```python
from build123d import *

# Parameters (mm, degrees)
F1_DEPTH       = 6.35
F2_R           = 3.81
F3_DEPTH       = 6.35
F5_D           = 1.9304
F5_CSINK_D     = 4.2672
F5_CSINK_ANGLE = 82
F7_D           = 2.032


with BuildPart() as f1:
    # F0 (on Front) → F1 (new body)
    with BuildSketch(Plane.XZ):
        with BuildLine():
            ThreePointArc((-5.08, 12.7), (-3.5921024484, 9.1078975516), (0, 7.62))
            Line((0, 7.62), (0, 12.7))
            Line((0, 12.7), (0, 17.78))
            ThreePointArc((0, 17.78), (-3.5921024484, 16.2921024484), (-5.08, 12.7))
        make_face()
        with BuildLine():
            Line((0, 12.7), (0, 7.62))
            ThreePointArc((0, 7.62), (3.5921024484, 9.1078975516), (5.08, 12.7))
            ThreePointArc((5.08, 12.7), (3.5921024484, 16.2921024484), (0, 17.78))
            Line((0, 17.78), (0, 12.7))
        make_face()
        with BuildLine():
            ThreePointArc((5.08, 12.7), (3.5921024484, 9.1078975516), (0, 7.62))
            ThreePointArc((0, 7.62), (-3.5921024484, 9.1078975516), (-5.08, 12.7))
            Line((-5.08, 12.7), (-5.08, 0))
            ThreePointArc((-5.08, 0), (0, -5.08), (5.08, 0))
            Line((5.08, 0), (5.08, 12.7))
        make_face()
        with BuildLine():
            ThreePointArc((0, 17.78), (3.5921024484, 16.2921024484), (5.08, 12.7))
            Line((5.08, 12.7), (5.08, 32.9050179497))
            Line((5.08, 32.9050179497), (4.3770618794, 31.711680915))
            ThreePointArc((4.3770618794, 31.711680915), (2.5207676458, 29.8795430536), (0, 29.21))
            Line((0, 29.21), (0, 17.78))
        make_face()
        with BuildLine():
            Line((-5.08, 34.29), (-5.08, 12.7))
            ThreePointArc((-5.08, 12.7), (-3.5921024484, 16.2921024484), (0, 17.78))
            Line((0, 17.78), (0, 29.21))
            ThreePointArc((0, 29.21), (-3.5921024484, 30.6978975516), (-5.08, 34.29))
        make_face()
        with BuildLine():
            Line((4.3770618794, 31.711680915), (5.08, 32.9050179497))
            Line((5.08, 32.9050179497), (5.08, 34.29))
            ThreePointArc((5.08, 34.29), (4.4104569464, 36.8107676458), (2.578319085, 38.6670618794))
            Line((2.578319085, 38.6670618794), (0, 34.29))
            Line((0, 34.29), (0, 29.21))
            ThreePointArc((0, 29.21), (2.5207676458, 29.8795430536), (4.3770618794, 31.711680915))
        make_face()
        with BuildLine():
            Line((5.08, 34.29), (5.08, 32.9050179497))
            Line((5.08, 32.9050179497), (25.0036145592, 66.7281759502))
            ThreePointArc((25.0036145592, 66.7281759502), (23.2048717648, 73.6835569145), (16.2494908004, 71.8848141201))
            Line((16.2494908004, 71.8848141201), (-4.3770618794, 36.868319085))
            ThreePointArc((-4.3770618794, 36.868319085), (-1.2719032275, 39.2081970456), (2.578319085, 38.6670618794))
            ThreePointArc((2.578319085, 38.6670618794), (4.4104569464, 36.8107676458), (5.08, 34.29))
        make_face()
        with BuildLine():
            ThreePointArc((-4.3770618794, 36.868319085), (-4.9011159111, 35.6262121188), (-5.08, 34.29))
            ThreePointArc((-5.08, 34.29), (-3.5921024484, 30.6978975516), (0, 29.21))
            Line((0, 29.21), (0, 34.29))
            Line((0, 34.29), (2.578319085, 38.6670618794))
            ThreePointArc((2.578319085, 38.6670618794), (-1.2719032275, 39.2081970456), (-4.3770618794, 36.868319085))
        make_face()
    extrude(amount=F1_DEPTH)

    # F2 (on face) → F3 (join)
    with BuildSketch(Plane.XZ.offset(6.35)):
        with Locations((0, 34.29)):
            Circle(F2_R)
    extrude(amount=F3_DEPTH)

    # F5 (through all)
    with Locations(Plane.XZ.offset(12.7)):
        with Locations((0, 34.29)):
            CounterSinkHole(F5_D / 2, F5_CSINK_D / 2, counter_sink_angle=F5_CSINK_ANGLE)

    # F7 (through all)
    with Locations(Plane.XZ.offset(6.35)):
        with Locations((0, 0)):
            Hole(F7_D / 2)


solid = f1.part
```
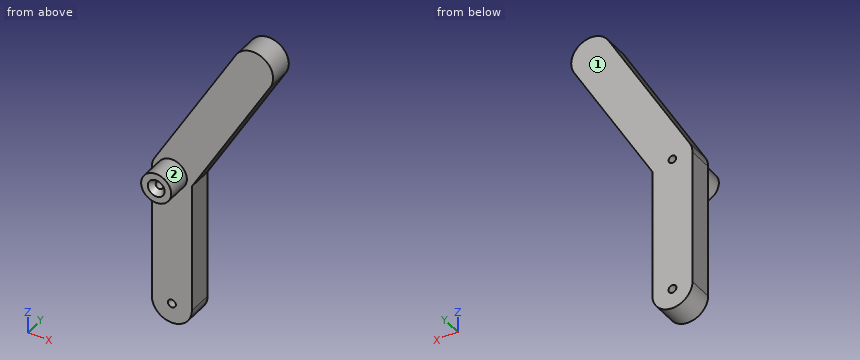
Here's how the part is built. I have some questions about the finished solid (model axes, mm). Face numbers are marked on the shaded views. A direction names the side the tool comes from. Coordinates: 2 decimals unless noted, no trailing zeros. Order: outer loops, then holes, each group sorted by start corner. A loop starts at its lowest first (then second) coordinate and runs counter-clockwise, first axis right, second up.
Item 1: I need wall thicknesses on probe 1 along Z at (x, y) = (0, -6); probe 2 along Z at (x, y) = (0, -7.25); probe 3 along X at (y, z) = (-3.5, 34.29). Which ranges of each line are inside material? Lowest first, please.
Response values:
probe 1: z = -5.08 to -1.02, 1.02 to 33.32, 35.26 to 44.3
probe 2: z = 30.48 to 33.32, 35.26 to 38.1
probe 3: x = -5.08 to -0.97, 0.97 to 5.9
Item 2: If we section it at D-D, the plane y = -9.75: List the corners of the cut face in (x, z) for me, then the cut area to 3 significant figures.
Response values:
outline: circle Ø7.62 at (0, 34.29); hole circle Ø1.93 at (0, 34.29)
area: 42.7 mm2
Item 3: If we section it at A-A, the plane x = 0: List the corners of the cut face in (y, z) for me.
Response values:
outline: (-12.7, 30.48) - (-6.35, 30.48) - (-6.35, 1.02) - (0, 1.02) - (0, 33.32) - (-11.36, 33.32) - (-12.7, 32.16) - close; (-12.7, 36.42) - (-11.36, 35.26) - (0, 35.26) - (0, 44.3) - (-6.35, 44.3) - (-6.35, 38.1) - (-12.7, 38.1) - close; (-6.35, -5.08) - (0, -5.08) - (0, -1.02) - (-6.35, -1.02) - close
Item 4: If we section it at B-B, the plane y = -2.25: List the corners of the cut face in (x, z) for me, then the cut area to 3 significant figures.
Response values:
outline: (-5.08, 0) arc R5.08 ccw to (5.08, 0) - (5.08, 32.91) - (25, 66.73) arc R5.08 ccw to (16.25, 71.88) - (-4.38, 36.87) arc R5.08 ccw to (-5.08, 34.29) - close; hole circle Ø2.03 at (0, 0); hole circle Ø1.93 at (0, 34.29)
area: 836 mm2
Item 5: I'm going to push flat-ended pins straight in: pin 1 Ø12 at (x, z) = (3.5, 21) entering from -Y; pin 2 Ø3 at (x, y) = (19, -5.5) entering from -Z; pin 3 Ø1.9 at (y, z) = (-4.5, 16) entering from +X; pin 4 Ø5 at (y, z) = (-11, 41) entering from +X. Where does each tip first touch, or does it pass through?
Response values:
pin 1: stops at y = -6.35
pin 2: stops at z = 53.99
pin 3: stops at x = 5.08
pin 4: passes through
Item 6: Which directions (+Z, -Z, +X, -X, +Y, -Y) give clear straight access to the entire face, cutting with the end or side of a thin tool? Please do the marked faces 1 and 2.
Response values:
face 1: +Z, -Z, +X, -X, +Y
face 2: -Y
Item 7: If we section it at C-C, the plane z = 8: List the corners of the cut face in (x, y) for me, then the cut area to 3 significant figures.
Response values:
outline: (-5.08, -6.35) - (5.08, -6.35) - (5.08, 0) - (-5.08, 0) - close
area: 64.5 mm2
